from build123d import *

# Parameters (mm, degrees)
CUT_EXTRUDE1_DEPTH = 4.7
SKETCH3_W          = 20
SKETCH3_H          = 20
CUT_EXTRUDE2_DEPTH = 2


with BuildPart() as part:
    # Sketch1 → Revolve1 (revolve)
    with BuildSketch(Plane(origin=(0, 0, 0), x_dir=(0, 0, -1), z_dir=(1, 0, 0))):
        with BuildLine():
            Line((-1.7, 0), (-1.7, 2))
            Line((-1.7, 2), (-12.9, 2))
            ThreePointArc((-12.9, 2), (-13.112132034, 2.087867966), (-13.2, 2.3))
            Line((-13.2, 2.3), (-12.770691475, 4.734729636))
            ThreePointArc((-12.770691475, 4.734729636), (-12.702287446, 4.853208889), (-12.573729924, 4.9))
            Line((-12.573729924, 4.9), (-11.4, 4.9))
            Line((-11.4, 4.9), (-11.4, 3.075))
            ThreePointArc((-11.4, 3.075), (-11.290165043, 2.809834957), (-11.025, 2.7))
            Line((-11.025, 2.7), (-10.6, 2.7))
            Line((-10.6, 2.7), (-10.6, 3.829289322))
            Line((-10.6, 3.829289322), (-10.529289322, 3.9))
            Line((-10.529289322, 3.9), (-10.3, 3.9))
            Line((-10.3, 3.9), (-10.3, 4))
            Line((-10.3, 4), (-0.7, 4))
            Line((-0.7, 4), (-0.7, 3.9))
            Line((-0.7, 3.9), (-0.6, 3.9))
            Line((-0.6, 3.9), (-0.5, 3.8))
            Line((-0.5, 3.8), (-0.4, 3.9))
            Line((-0.4, 3.9), (0, 3.9))
            Line((0, 3.9), (0, 2.5))
            Line((0, 2.5), (2.5095, 2.5))
            Line((2.5095, 2.5), (3, 2.0095))
            Line((3, 2.0095), (3, 0))
            Line((3, 0), (-1.7, 0))
        make_face()
    revolve(axis=Axis((0, 0, -3), (0, 0, 1)))

    # Sketch2 → Cut-Extrude1 (cut)
    with BuildSketch(Plane.XY.offset(-3)):
        Polygon((-1.25, -0.721687836), (0, -1.443375673), (1.25, -0.721687836), (1.25, 0.721687836), (0, 1.443375673), (-1.25, 0.721687836), align=None)
    extrude(amount=CUT_EXTRUDE1_DEPTH, mode=Mode.SUBTRACT)

    # Sketch3 → Cut-Extrude2 (cut)
    with BuildSketch(Plane.XY.offset(13.2)):
        Rectangle(SKETCH3_W, SKETCH3_H)
        with BuildLine():
            Line((-3.9, 1), (-3.9, -1))
            ThreePointArc((-3.9, -1), (0, -4.899999854), (3.9, -1))
            Line((3.9, -1), (3.9, 1))
            ThreePointArc((3.9, 1), (0, 4.9), (-3.9, 1))
        make_face(mode=Mode.SUBTRACT)
    extrude(amount=-CUT_EXTRUDE2_DEPTH, mode=Mode.SUBTRACT)


solid = part.part
Part model, mm, in its own coordinate system. A direction names the side the tool comes from. Round coordinates to 2 decimals unless told otherwise and drop trailing zeros. Write each loop counter-clockwise with the first axis right and the second up, starting at its lowest first coordinate (ties: lowest second). Pieces come first, ordered by that corner, then holes. Notation, with made-up numbers: (-16.75, -30) - (24.25, -30) arc R32 ccw to (24.25, 1) - close; hole circle Ø11 at (65, 35). An arc over 180 degrees is marked (long way). Use CSV: the item, a comma, the result in double quotes.
Item 1: Tool access for faces 1 (the flat face through (1, 3, 10.6)), 2 (the cylindrical face through (3.905, -0.867, 5.433)), 3 (the flat face through (-1.25, 0, -1)): list every direction of +Z, -Z, +X, -X, +Y, -Y with a clear straight run to the whole face (end or side of a thin tool).
Results list:
face 1,"none"
face 2,"-Z"
face 3,"+Z, -Z"
Item 2: Slice it at A-A, the plane z = -1.25. Write the cut outline in (x, y), then the cut area to 3 significant figures.
Results list:
outline,"circle Ø5 at (0, 0); hole (-1.25, -0.72) - (0, -1.44) - (1.25, -0.72) - (1.25, 0.72) - (0, 1.44) - (-1.25, 0.72) - close"
area,"14.2 mm²"
Item 3: Wall check: L1, parallel to Y at x = 0, z = 7.25; L2, parallel to Z at x = 3.75, y = -1.5. Give the ranges that are in metal, low to high.
Results list:
L1,"y = -4 to -2, 2 to 4"
L2,"z = 11.4 to 12.89"
Item 4: Pull direction X, two halves, no side cores. Call faces 4 (the cylindrical face through (2.44, -0.54, -1.27)), 5 (the flat face through (-0.1, -3.3, 11.4)), 6 (the flat face through (-0.63, -1.08, -0.68)): pulls with the +X half, pulls with the -X half, needs draft (parallel to the pull), parting line crosses it, or undercut.
Results list:
face 4,"parting line crosses it"
face 5,"needs draft"
face 6,"undercut"
Item 5: Flat gauge pins, fed straight in: P1, Ø0.7, axis at y = 0.5, z = -1, coming from the +X side; P2, Ø1.2, axis at x = -0.5, y = 1, coming from the +Z side; P3, Ø1.2, axis at y = -0.5, z = -1, coming from the -X side; P4, Ø1, axis at x = -0.5, y = -0.5, coming from the +Z side. Where does each tip first touch, or does it go through?
Results list:
P1,"stops at x = 2.5"
P2,"stops at z = 1.7"
P3,"stops at x = -2.5"
P4,"passes through"
Item 6: Slice it at B-B, the plane z = 4.5. Write the cut outline in (x, y).
Results list:
outline,"circle Ø8 at (0, 0); hole circle Ø4 at (0, 0)"
